Job drawing, mm, ordinate dimensions from the low corner. One solid piece. Coordinates: 2 decimals unless noted, no trailing zeros. Loops run counter-clockwise (first coordinate to the right, second up) from the corner with the lowest first, then second, coordinate; pieces in that order, holes last. Notation, with made-up numbers: M 46,-16 L 60,-16 A7 cw 60,-6 Z; hole C 57,66 d4. An arc over 180 degrees is marked long. Answer as a JSON object with one key per item and string values. Group by question number.
1. Drop flat-ended pins along their axis: pin 1 Ø3 at (x, z) = (117, 17.5) entering from -Y; pin 2 Ø6 at (x, z) = (122, 21) entering from +Y; pin 3 Ø3 at (x, z) = (179, 9.5) entering from -Y. Give the stop position or say it passes through.
2. Drill centre lines: L1, parallel to Y at x = 222, z = 29.25; L2, parallel to Y at x = 179.5, z = 19.5. Where is each one in solid material? Low to high.
3. Saw through at A-A on x = 35.5. Write the cut outline in (y, z), then the cut area to 4 significant figures.
4. Saw through at B-B on z = 7.5. Write the cut outline in (x, y), then the cut area to 4 significant figures.
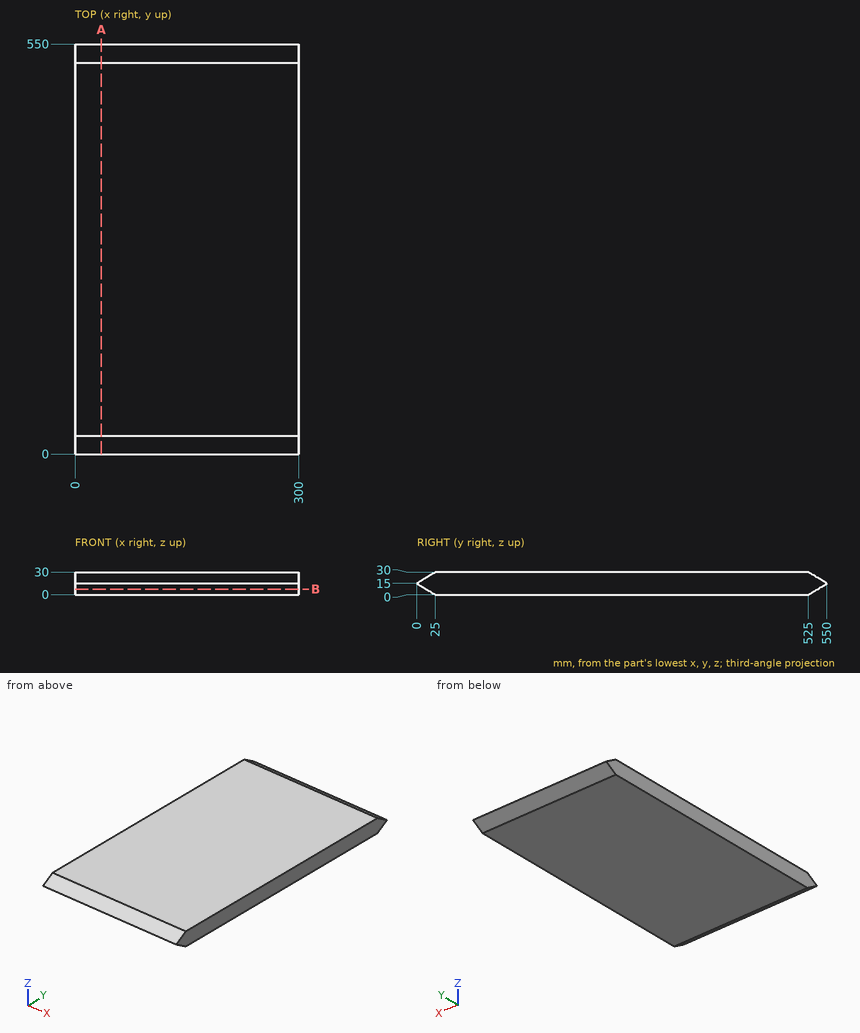
Outcome:
{
 "1": {"pin 1": "stops at y = 1.67", "pin 2": "stops at y = 545", "pin 3": "stops at y = 6.67"},
 "2": {"L1": "y = 23.75 to 526.25", "L2": "y = 7.5 to 542.5"},
 "3": {"outline": "M 0,15 L 25,0 L 525,0 L 550,15 L 525,30 L 25,30 Z", "area": "15,750 mm²"},
 "4": {"outline": "M 0,12.5 L 300,12.5 L 300,537.5 L 0,537.5 Z", "area": "157,500 mm²"}
}
